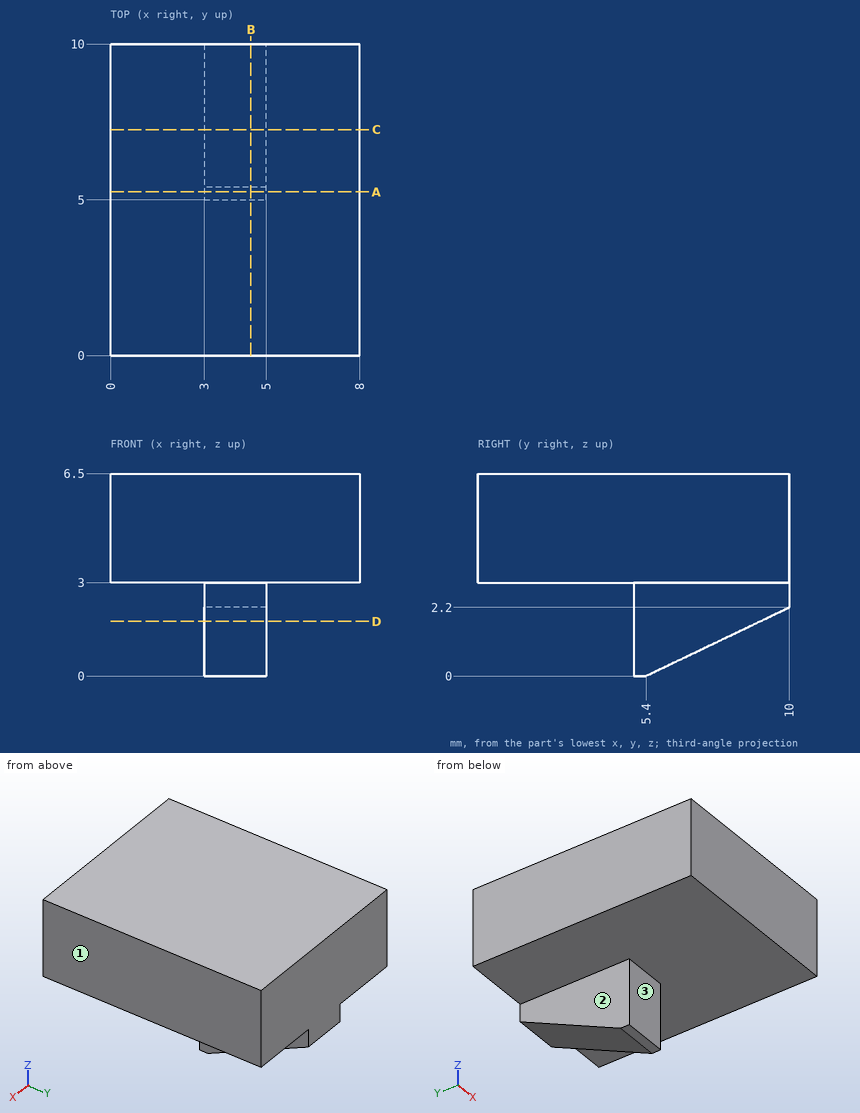
The drawing under review shows one solid part. Ordinate dimensions are in mm from its lowest x, y, z. A direction names the side the tool comes from. Round coordinates to 2 decimals unless told otherwise and drop trailing zeros. Loops run counter-clockwise (first coordinate to the right, second up) from the corner with the lowest first, then second, coordinate; pieces in that order, holes last. Notation, with made-up numbers: (68, 45.25) -> (98, 45.25) arc R21 ccw to (98, 66.25) -> close; hole circle Ø1 at (-12.5, 42). An arc over 180 degrees is marked (long way). One line per question, with ' | ' between items. Start each with the question number.
Item 1: For pin 1 (3 mm diameter, centred on x = 4, y = 6.5, fed in from -Z); pin 2 (1.5 mm diameter, centred on y = 8.5, z = 2, fed in from -X); pin 3 (3.5 mm diameter, centred on y = 8, z = 1, fed in from +X); pin 4 (1 mm diameter, centred on x = 3.5, z = 1.5, fed in from -Y), all flat-tipped, find the tip position at first contact; note any pin that passes through.
Item 2: Add section D-D, the plane z = 1.75. Write out the cut boundary in (x, y), then the cut area to 3 significant figures.
Item 3: Wall thickness on line 1 along X through (y, z) = (6.25, 1.5); line 2 along Z through (x, y) = (2, 5.5); line 3 along Z through (x, y) = (3.75, 7.25): over which ranges is each line inside the solid? List them lowest first. Write a range as [from, to].
Item 4: Add section A-A, the plane y = 5.25. Write out the cut boundary in (x, z).
Item 5: Add section C-C, the plane y = 7.25. Write out the cut boundary in (x, z).
Item 6: Add section B-B, the plane x = 4.5. Write out the cut boundary in (y, z), then the cut area to 3 significant figures.
Item 7: Machinability: for the marked faces 1, 2 and 3, which of the approach directions +Z, -Z, +X, -X, +Y, -Y give a long, thin tool a straight path to every point of the face, cutting with its end or side? Answer none if there is none.
Return value:
1) pin 1: stops at z = 0 | pin 2: stops at x = 3 | pin 3: stops at x = 5 | pin 4: stops at y = 5
2) outline: (3, 5) -> (5, 5) -> (5, 9.06) -> (3, 9.06) -> close | area: 8.12 mm2
3) line 1: x = [3, 5] | line 2: z = [3, 6.5] | line 3: z = [0.88, 6.5]
4) outline: (0, 3) -> (3, 3) -> (3, 0) -> (5, 0) -> (5, 3) -> (8, 3) -> (8, 6.5) -> (0, 6.5) -> close
5) outline: (0, 3) -> (3, 3) -> (3, 0.88) -> (5, 0.88) -> (5, 3) -> (8, 3) -> (8, 6.5) -> (0, 6.5) -> close
6) outline: (0, 3) -> (5, 3) -> (5, 0) -> (5.4, 0) -> (10, 2.2) -> (10, 6.5) -> (0, 6.5) -> close | area: 44.9 mm2
7) face 1: +Z, -Z, +X, +Y, -Y | face 2: -Z, -X, +Y, -Y | face 3: -Z, +X, -X, -Y
